Verification items for the finished model (mm, model axes). Face numbers are marked on the shaded views. Round coordinates to 2 decimals unless told otherwise and drop trailing zeros. Loops run counter-clockwise (first coordinate to the right, second up) from the corner with the lowest first, then second, coordinate; pieces in that order, holes last. Notation, with made-up numbers: M 67,-16 L 84,-16 A20 ccw 84,0 Z; hole C -12,6 d7. An arc over 180 degrees is marked long. Answer as CSV lines item,"result".
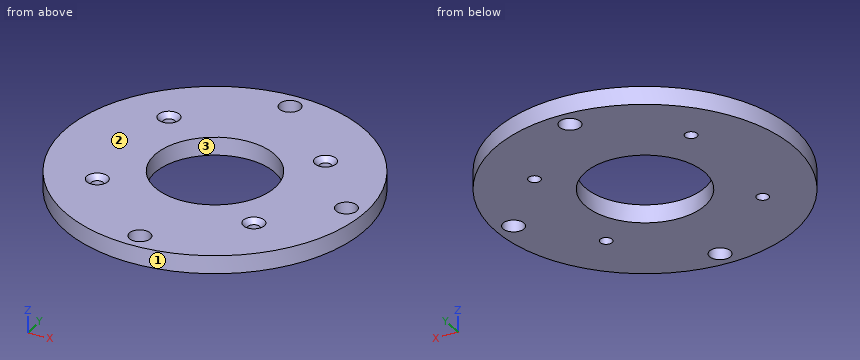
```python
from build123d import *

# Parameters (mm, degrees)
SKETCH_1_W          = 25
SKETCH_1_H          = 3
HOLE_WIZARD_1_D     = 2.013
HOLE_WIZARD_2_D     = 2.013
HOLE_WIZARD_2_DEPTH = 3
HOLE_WIZARD_3_D     = 2.013
HOLE_WIZARD_3_DEPTH = 3
HOLE_WIZARD_4_D     = 2.013
HOLE_WIZARD_4_DEPTH = 3
HOLE_WIZARD_5_D     = 3.5
HOLE_WIZARD_5_DEPTH = 3
HOLE_WIZARD_6_D     = 3.5
HOLE_WIZARD_6_DEPTH = 3
HOLE_WIZARD_7_D     = 20
HOLE_WIZARD_7_DEPTH = 3
HOLE_WIZARD_8_D     = 3.5
HOLE_WIZARD_8_DEPTH = 3
CHAMFER_1_SIZE      = 0.7435
CHAMFER_1_SIZE2     = 0.855298911
CHAMFER_2_SIZE      = 0.7435
CHAMFER_2_SIZE2     = 0.855298911
CHAMFER_3_SIZE      = 0.7435
CHAMFER_3_SIZE2     = 0.855298911
CHAMFER_4_SIZE      = 0.7435
CHAMFER_4_SIZE2     = 0.855298911


with BuildPart() as part:
    # Эскиз1 → Повернуть1 (revolve)
    with BuildSketch(Plane(origin=(0, 0, 0), x_dir=(1, 0, 0), z_dir=(0, 1, 0))):
        with Locations((12.5, -1.5)):
            Rectangle(SKETCH_1_W, SKETCH_1_H)
    revolve(axis=Axis((0, 0, 0), (0, 0, 1)))

    # Отверстие1 (through all)
    with Locations(Plane.XY.offset(3)):
        with Locations((-13.7, -10.5)):
            Hole(HOLE_WIZARD_1_D / 2)

    # Отверстие2
    with Locations(Plane.XY.offset(3)):
        with Locations((12.5, 10.5)):
            Hole(HOLE_WIZARD_2_D / 2, depth=HOLE_WIZARD_2_DEPTH)

    # Отверстие3
    with Locations(Plane.XY.offset(3)):
        with Locations((-13.7, 10.5)):
            Hole(HOLE_WIZARD_3_D / 2, depth=HOLE_WIZARD_3_DEPTH)

    # Отверстие4
    with Locations(Plane.XY.offset(3)):
        with Locations((12.5, -10.5)):
            Hole(HOLE_WIZARD_4_D / 2, depth=HOLE_WIZARD_4_DEPTH)

    # Отверстие5
    with Locations(Plane.XY.offset(3)):
        with Locations((0, -22)):
            Hole(HOLE_WIZARD_5_D / 2, depth=HOLE_WIZARD_5_DEPTH)

    # Отверстие6
    with Locations(Plane.XY.offset(3)):
        with Locations((0, 22)):
            Hole(HOLE_WIZARD_6_D / 2, depth=HOLE_WIZARD_6_DEPTH)

    # Отверстие7
    with Locations(Plane.XY.offset(3)):
        with Locations((0, 0)):
            Hole(HOLE_WIZARD_7_D / 2, depth=HOLE_WIZARD_7_DEPTH)

    # Отверстие8
    with Locations(Plane.XY.offset(3)):
        with Locations((22, 0)):
            Hole(HOLE_WIZARD_8_D / 2, depth=HOLE_WIZARD_8_DEPTH)

    # Фаска1
    chamfer_1_edges = [part.edges().sort_by_distance(p)[0] for p in [
        (-12.6935, 10.5, 3),
    ]]
    chamfer_1_side = [part.faces().sort_by_distance(p)[0] for p in [
        (-24.292893219, 0, 3),
    ]]
    chamfer(chamfer_1_edges, length=CHAMFER_1_SIZE, length2=CHAMFER_1_SIZE2, reference=chamfer_1_side[0])

    # Фаска2
    chamfer_2_edges = [part.edges().sort_by_distance(p)[0] for p in [
        (13.5065, -10.5, 3),
    ]]
    chamfer_2_side = [part.faces().sort_by_distance(p)[0] for p in [
        (-11.242893219, 10.5, 3),
    ]]
    chamfer(chamfer_2_edges, length=CHAMFER_2_SIZE, length2=CHAMFER_2_SIZE2, reference=chamfer_2_side[0])

    # Фаска3
    chamfer_3_edges = [part.edges().sort_by_distance(p)[0] for p in [
        (13.5065, 10.5, 3),
    ]]
    chamfer_3_side = [part.faces().sort_by_distance(p)[0] for p in [
        (14.957106781, -10.5, 3),
    ]]
    chamfer(chamfer_3_edges, length=CHAMFER_3_SIZE, length2=CHAMFER_3_SIZE2, reference=chamfer_3_side[0])

    # Фаска4
    chamfer_4_edges = [part.edges().sort_by_distance(p)[0] for p in [
        (-12.6935, -10.5, 3),
    ]]
    chamfer_4_side = [part.faces().sort_by_distance(p)[0] for p in [
        (14.957106781, 10.5, 3),
    ]]
    chamfer(chamfer_4_edges, length=CHAMFER_4_SIZE, length2=CHAMFER_4_SIZE2, reference=chamfer_4_side[0])


solid = part.part
```
1) Go/stop test with flat-tipped pins: pin 1 (1 mm diameter, centred on x = -20, y = -16, fed in from +Z); pin 2 (2.5 mm diameter, centred on x = -13.7, y = 10.5, fed in from +Z); pin 3 (1 mm diameter, centred on y = -5.5, z = 2, fed in from -X); pin 4 (3 mm diameter, centred on x = 12.5, y = -10.5, fed in from +Z). Record where each tip stops, or that it passes through.
Here are the results:
pin 1,"passes through"
pin 2,"stops at z = 2.42"
pin 3,"stops at x = -24.49"
pin 4,"stops at z = 2.71"
2) Section check B-B (y = 0). Record the cut outline in (x, z), plus the area to 3 significant figures.
Here are the results:
outline,"M -25,0 L -10,0 L -10,3 L -25,3 Z; M 10,0 L 20.25,0 L 20.25,3 L 10,3 Z; M 23.75,0 L 25,0 L 25,3 L 23.75,3 Z"
area,"79.5 mm^2"
3) Section check A-A (z = 1.1). State how many separate pieces and enclosed holes the cut face has, plus the area to 3 significant figures.
Here are the results:
separate pieces,"1"
enclosed holes,"8"
area,"1,610 mm^2"
4) Material ranges on probe 1 along Y at (x, z) = (0, 0.3); probe 2 along Y at (x, z) = (-13.5, 2.7); probe 3 along X at (y, z) = (9, 1.85), recorded low to high.
Here are the results:
probe 1,"y = -25 to -23.75, -20.25 to -10, 10 to 20.25, 23.75 to 25"
probe 2,"y = -21.04 to -11.98, -9.02 to 9.02, 11.98 to 21.04"
probe 3,"x = -23.32 to -4.36, 4.36 to 23.32"
5) Section check C-C (x = -4). Record the cut outline in (y, z).
Here are the results:
outline,"M -24.68,0 L -9.17,0 L -9.17,3 L -24.68,3 Z; M 9.17,0 L 24.68,0 L 24.68,3 L 9.17,3 Z"
6) Draft check along X on the marked faces 1, 2 and 3. Enter one of: +X half, -X half, draft (parallel to the pull), parting line (faces both ways), or undercut.
Here are the results:
face 1,"parting line"
face 2,"draft"
face 3,"undercut"
7) Section check D-D (x = 12.5). Record the cut outline in (y, z), plus the area to 3 significant figures.
Here are the results:
outline,"M -21.65,0 L -11.51,0 L -11.51,2.14 L -12.25,3 L -21.65,3 Z; M -9.49,0 L 9.49,0 L 9.49,2.14 L 8.75,3 L -8.75,3 L -9.49,2.14 Z; M 11.51,0 L 21.65,0 L 21.65,3 L 12.25,3 L 11.51,2.14 Z"
area,"117 mm^2"
